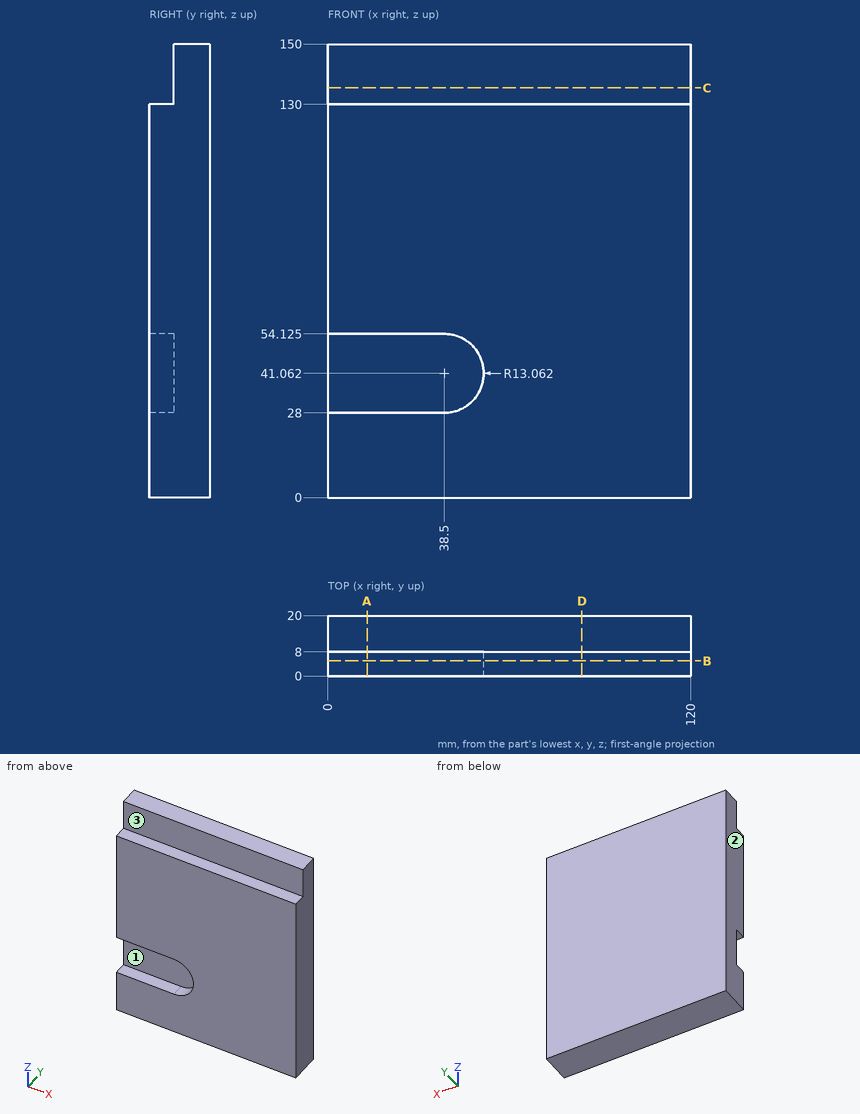
Source: three-view drawing plus pictorial views. Frame: mm from the lowest corner of the part. A direction names the side the tool comes from. Coordinates: 2 decimals unless noted, no trailing zeros. Loops run counter-clockwise (first coordinate to the right, second up) from the corner with the lowest first, then second, coordinate; pieces in that order, holes last. Notation, with made-up numbers: (-1.75, 62.5) - (56.25, 62.5) arc R7 cw to (56.25, 74.5) - close; hole circle Ø10 at (40, 64.5). An arc over 180 degrees is marked (long way). One line per item, written item: value. Start each with the question number.
1. Set-up query: the marked faces 1, 2 and 3. Return all of +Z, -Z, +X, -X, +Y, -Y with unobstructed straight access to the full face (end or side cutting, diameter ignored); none if empty.
2. Section B-B (y = 5). Return the cut outline in (x, z) (1 decimal).
3. Section A-A (x = 13). Return the cut outline in (y, z) (1 decimal), and give its area (3 significant figures).
4. Ray query, L1, parallel to Z at x = 24.5, y = 5.5 (1 decimal); L2, parallel to Z at x = 60, y = 3.5; L3, parallel to X at y = 5.75, z = 49.5. Return the intervals inside material, ascending.
5. Section C-C (z = 135.5). Return the cut outline in (x, y), and give its area (3 significant figures).
6. Contact query for flat-ended pins moving along their axis: P1, Ø2.5, axis at x = 44.5, y = 3.5, coming from the +Z side; P2, Ø10, axis at x = 60.5, z = 138.5, coming from the -Y side. Output: stop coordinate, or through.
7. Section D-D (x = 84). Return the cut outline in (y, z).
Verdict:
1. face 1: -X, -Y
1. face 2: +Z, -Z, -X, +Y, -Y
1. face 3: +Z, +X, -X, -Y
2. outline: (0, 0) - (120, 0) - (120, 130) - (0, 130) - (0, 54.1) - (38.5, 54.1) arc R13.1 cw to (38.5, 28) - (0, 28) - close
3. outline: (0, 0) - (20, 0) - (20, 150) - (8, 150) - (8, 130) - (0, 130) - (0, 54.1) - (8, 54.1) - (8, 28) - (0, 28) - close
3. area: 2,630 mm2
4. L1: z = 0 to 28, 54.1 to 130
4. L2: z = 0 to 130
4. L3: x = 48.47 to 120
5. outline: (0, 8) - (120, 8) - (120, 20) - (0, 20) - close
5. area: 1,440 mm2
6. P1: stops at z = 130
6. P2: stops at y = 8
7. outline: (0, 0) - (20, 0) - (20, 150) - (8, 150) - (8, 130) - (0, 130) - close
